Source: CAD feature listing. Evaluate the final solid. Frame: model axes, mm. Face numbers are marked on the shaded views. A direction names the side the tool comes from. Coordinates: 2 decimals unless noted, no trailing zeros. Write each loop counter-clockwise with the first axis right and the second up, starting at its lowest first coordinate (ties: lowest second). Pieces come first, ordered by that corner, then holes. Notation, with made-up numbers: M 77,25.5 L 84,25.5 A12 ccw 84,44.5 Z; hole C 73,1.5 d11. An arc over 180 degrees is marked long. Answer as CSV lines item,"result". Start each with the question number.
1. Mould query, pull axis X, two halves, no side actions, for the marked faces 1, 2 and 3. Classes: pulls with the +X half, pulls with the -X half, needs draft (parallel to the pull), parting line crosses it, or undercut.
2. Section A-A on x = 58.5. Return the cut outline in (y, z), plus the area to 3 significant figures.
3. Contact query for flat-ended pins moving along their axis: pin 1 Ø1.5 at (y, z) = (-4, -1.5) entering from +X; pin 2 Ø4 at (x, z) = (92, 0) entering from -Y; pin 3 Ø1.5 at (x, z) = (32, -1.5) entering from +Y. Output: stop coordinate, or through.
4. Line query: probe 1 along X at (y, z) = (-3.75, -6); probe 2 along X at (y, z) = (-2.5, 3.5); probe 3 along Z at (x, y) = (72, -2.75). Output: solid intervals per line, ascending. Write a range as [from, to].
5. Reachability of the marked faces 4, 5, 6, 7 and 8 from +Z, -Z, +X, -X, +Y, -Y: full face, straight path, thin tool, end or side. Return the list, or none.
```python
from build123d import *

# Parameters (mm, degrees)
CUT_EXTRUDE8_DEPTH = 10
CUT_EXTRUDE9_DEPTH = 10


with BuildPart() as part:
    # Sketch3 → Revolve1 (revolve)
    with BuildSketch(Plane(origin=(0, 0, 0), x_dir=(1, 0, 0), z_dir=(0, 1, 0)), mode=Mode.PRIVATE) as revolve1_sk:
        Polygon((0, 0), (113.3, 0), (113.3, 4.99), (39.5, 4.99), (39.5, 4.79), (38.5, 4.79), (38.5, 4.99), (30.5, 4.99), (30.5, 4.79), (29.5, 4.79), (29.5, 4.99), (26, 4.99), (26, 7.49), (14, 7.49), (14, 4.99), (4, 4.99), (4, 4.79), (3, 4.79), (3, 4.99), (0, 4.99), align=None)
    revolve(revolve1_sk.sketch.rotate(Axis((0, 0, 0), (1, 0, 0)), 180), axis=Axis((0, 0, 0), (1, 0, 0)))

    # Sketch10 → Cut-Extrude8 (cut)
    with BuildSketch(Plane.ZY.offset(-14)):
        with BuildLine():
            Line((7.228416147, 2), (-7.228416147, 2))
            ThreePointArc((-7.228416147, 2), (0, 7.5), (7.228416147, 2))
        make_face()
        with BuildLine():
            Line((7.228416147, -2), (-7.228416147, -2))
            ThreePointArc((-7.228416147, -2), (0, -7.5), (7.228416147, -2))
        make_face()
    extrude(amount=-CUT_EXTRUDE8_DEPTH, mode=Mode.SUBTRACT)

    # Sketch11 → Cut-Extrude9 (cut)
    with BuildSketch(Plane(origin=(113.3, 0, 0), x_dir=(0, 0, -1), z_dir=(1, 0, 0))):
        with BuildLine():
            Line((-4.582575695, -2), (4.582575695, -2))
            ThreePointArc((4.582575695, -2), (0, -5), (-4.582575695, -2))
        make_face()
        with BuildLine():
            Line((4.582575695, 2), (-4.582575695, 2))
            ThreePointArc((-4.582575695, 2), (0, 5), (4.582575695, 2))
        make_face()
    extrude(amount=-CUT_EXTRUDE9_DEPTH, mode=Mode.SUBTRACT)


solid = part.part
```
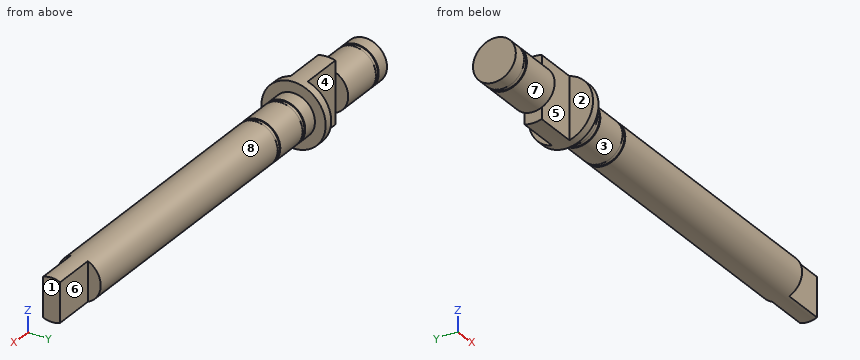
Values:
1,face 1,"pulls with the +X half"
1,face 2,"undercut"
1,face 3,"needs draft"
2,outline,"C 0,0 d9.98"
2,area,"78.2 mm²"
3,pin 1,"x = 103.3"
3,pin 2,"y = -4.99"
3,pin 3,"y = 4.93"
4,probe 1,"[24, 26]"
4,probe 2,"[0, 14], [24, 103.3]"
4,probe 3,"[-4.16, 4.16]"
5,face 4,"+Z, -Z, +Y"
5,face 5,"+Z, -Z, -Y"
5,face 6,"+Z, -Z, +X, +Y"
5,face 7,"-X"
5,face 8,"+X"
